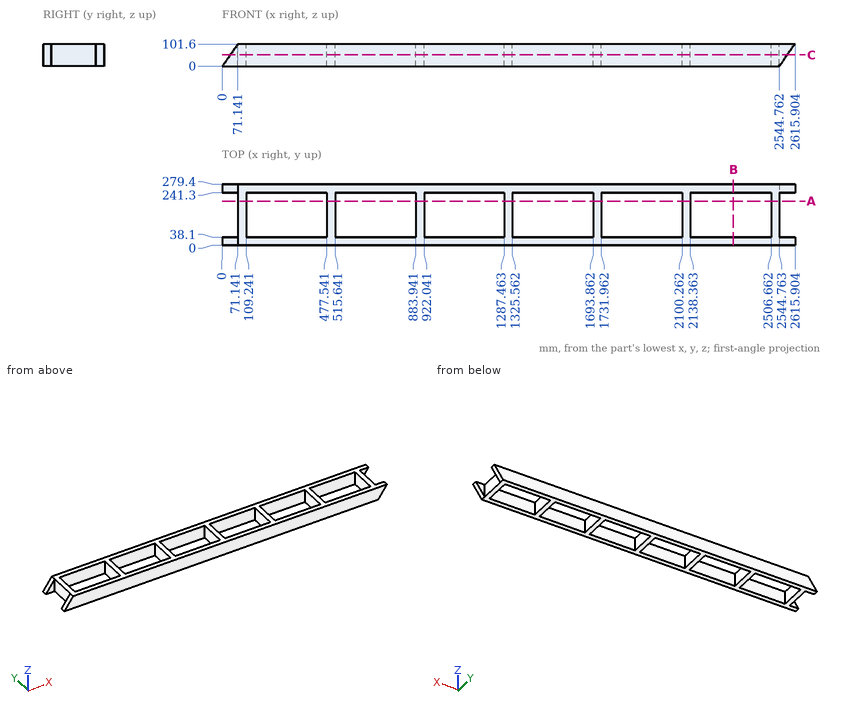
Could you check a few things on this drawing? It's one solid part, dimensions in mm from its lowest x, y, z. Coordinates: 2 decimals unless noted, no trailing zeros. Write each loop counter-clockwise with the first axis right and the second up, starting at its lowest first coordinate (ties: lowest second). Pieces come first, ordered by that corner, then holes. Notation, with made-up numbers: (-15.75, 16) - (33.25, 16) arc R23 cw to (33.25, 49) - close; hole circle Ø4 at (4.5, -18). An arc over 180 degrees is marked (long way). Write item = value, one per line.
1) Suppose I cut it at A-A on y = 202.5. Please give me the cut outline in (x, z).
Result set:
outline = (71.14, 0) - (109.24, 0) - (109.24, 101.6) - (71.14, 101.6) - close; (477.54, 0) - (515.64, 0) - (515.64, 101.6) - (477.54, 101.6) - close; (883.94, 0) - (922.04, 0) - (922.04, 101.6) - (883.94, 101.6) - close; (1287.46, 0) - (1325.56, 0) - (1325.56, 101.6) - (1287.46, 101.6) - close; (1693.86, 0) - (1731.96, 0) - (1731.96, 101.6) - (1693.86, 101.6) - close; (2100.26, 0) - (2138.36, 0) - (2138.36, 101.6) - (2100.26, 101.6) - close; (2506.66, 0) - (2544.76, 0) - (2544.76, 101.6) - (2506.66, 101.6) - close
2) Please list where these lines run through material, in increasing order: line 1 (Y direction, x = 2264, z = 74); line 2 (X direction, y = 243, z = 40); line 3 (X direction, y = 245.5, z = 86). Write a range as [from, to].
Result set:
line_1 = [0, 38.1], [241.3, 279.4]
line_2 = [28.01, 2572.77]
line_3 = [60.22, 2604.98]
3) Suppose I cut it at C-C on z = 51.5. State how many separate pieces and enclosed holes the cut face has, plus the area to 3 significant figures.
Result set:
separate_pieces = 1
enclosed_holes = 6
area = 248,000 mm2
4) Will these pins go through, and if not, where does the flat tip stop? pin 1 Ø12 at (y, z) = (126.5, 71.5) entering from +X; pin 2 Ø5 at (x, z) = (1889, 33) entering from -Y; pin 3 Ø10 at (y, z) = (86.5, 74) entering from -X.
Result set:
pin_1 = 2544.76
pin_2 = 0
pin_3 = 71.14
5) Suppose I cut it at B-B on x = 2335. Please give me the cut outline in (y, z).
Result set:
outline = (0, 0) - (38.1, 0) - (38.1, 101.6) - (0, 101.6) - close; (241.3, 0) - (279.4, 0) - (279.4, 101.6) - (241.3, 101.6) - close
